Part model, mm, in its own coordinate system. A direction names the side the tool comes from. Round coordinates to 2 decimals unless told otherwise and drop trailing zeros. Answer as a JSON object with one key per item and string values. Group by question number.
1. Drop flat-ended pins along their axis: pin 1 (0.6 mm diameter, centred on x = 3, z = -4, fed in from +Y); pin 2 (0.6 mm diameter, centred on x = -3.5, z = 4, fed in from -Y); pin 3 (0.6 mm diameter, centred on y = -9, z = -4, fed in from -X). Give the stop position or say it passes through.
2. Drill centre lines: line 1 (Y direction, x = 0, z = 3.95); line 2 (X direction, y = 5, z = 3.75); line 3 (Y direction, x = -7.5, z = 4). Where is each one in solid material? Low to high. Write a range as from..to.
3. Which spindle directions (+Z, -Z, +X, -X, +Y, -Y) get a long thin tool onto all of the face, cutting with end or side? Do faces 1 (the face through (-27.49, -55.69, -3.9)), 2 (the face through (-27.39, 55.79, -3.9)), 3 (the face through (-27.49, -55.69, 3.9)), 4 (the face through (27.39, -55.79, -3.9)), 5 (the face through (27.49, 55.69, 3.9)). Say none if no direction does.
from build123d import *

# Parameters (mm, degrees)
F1_DEPTH = 4.65
F3_DEPTH = 3.65
F4_SIZE  = 0.5
F5_SIZE  = 0.5
F6_SIZE  = 0.5
F7_SIZE  = 0.5
F9_D     = 10
F9_DEPTH = 1
F9_TIP   = 3.0043030951


with BuildPart() as f1:
    # F0 (on Top) → F1 (new body, symmetric)
    with BuildSketch(Plane.XY):
        with BuildLine():
            Line((-22.95, -57.6), (22.95, -57.6))
            ThreePointArc((22.95, -57.6), (27.4401280605, -55.7401280605), (29.3, -51.25))
            Line((29.3, -51.25), (29.3, 51.25))
            ThreePointArc((29.3, 51.25), (27.4401280605, 55.7401280605), (22.95, 57.6))
            Line((22.95, 57.6), (-22.95, 57.6))
            ThreePointArc((-22.95, 57.6), (-27.4401280605, 55.7401280605), (-29.3, 51.25))
            Line((-29.3, 51.25), (-29.3, -51.25))
            ThreePointArc((-29.3, -51.25), (-27.4401280605, -55.7401280605), (-22.95, -57.6))
        make_face()
    extrude(amount=F1_DEPTH, both=True)

    # F2 (on Top) → F3 (join, symmetric)
    with BuildSketch(Plane.XY):
        with BuildLine():
            Line((-23.95, -58.6), (23.95, -58.6))
            ThreePointArc((23.95, -58.6), (28.4401280605, -56.7401280605), (30.3, -52.25))
            Line((30.3, -52.25), (30.3, 52.25))
            ThreePointArc((30.3, 52.25), (28.4401280605, 56.7401280605), (23.95, 58.6))
            Line((23.95, 58.6), (-23.95, 58.6))
            ThreePointArc((-23.95, 58.6), (-28.4401280605, 56.7401280605), (-30.3, 52.25))
            Line((-30.3, 52.25), (-30.3, -52.25))
            ThreePointArc((-30.3, -52.25), (-28.4401280605, -56.7401280605), (-23.95, -58.6))
        make_face()
    extrude(amount=F3_DEPTH, both=True)

    # F4
    f4_edges = [f1.edges().sort_by_distance(p)[0] for p in [
        (-30.3, 0, 3.65),
    ]]
    chamfer(f4_edges, length=F4_SIZE)

    # F5
    f5_edges = [f1.edges().sort_by_distance(p)[0] for p in [
        (-30.3, 0, -3.65),
    ]]
    chamfer(f5_edges, length=F5_SIZE)

    # F6
    f6_edges = [f1.edges().sort_by_distance(p)[0] for p in [
        (-29.3, 0, 4.65),
    ]]
    chamfer(f6_edges, length=F6_SIZE)

    # F7
    f7_edges = [f1.edges().sort_by_distance(p)[0] for p in [
        (29.3, 0, -4.65),
    ]]
    chamfer(f7_edges, length=F7_SIZE)

    # F9
    with Locations(Plane.XY.offset(4.65)):
        with Locations((0, -50.1860789955)):
            Hole(F9_D / 2, depth=F9_DEPTH)
            with Locations((0, 0, -(F9_DEPTH + F9_TIP / 2))):  # 118° drill point
                Cone(0, F9_D / 2, F9_TIP, mode=Mode.SUBTRACT)


solid = f1.part
Worked answers:
{
 "1": {"pin 1": "stops at y = 57.6", "pin 2": "stops at y = -57.6", "pin 3": "stops at x = -29.3"},
 "2": {"line 1": "y = -57.6..-55.19, -45.19..57.6", "line 2": "x = -29.3..29.3", "line 3": "y = -57.6..57.6"},
 "3": {"face 1": "-Z, -X, -Y", "face 2": "-Z, -X, +Y", "face 3": "+Z, -X, -Y", "face 4": "-Z, +X, -Y", "face 5": "+Z, +X, +Y"}
}
